Check sheet for the modelled part. Datum: model origin and axes. Units: mm. Face numbers are marked on the shaded views. Round coordinates to 2 decimals unless told otherwise and drop trailing zeros. Order: outer loops, then holes, each group sorted by start corner. A loop starts at its lowest first (then second) coordinate and runs counter-clockwise, first axis right, second up.
Q1. Cross-section at D-D on y = 2.5. Give the number of separate pieces and of enclosed holes in the cut face, then the cut area to 3 significant figures.
Q2. Cross-section at B-B on z = 9. Record the cut outline in (x, y), then the cut area to 3 significant figures.
Q3. Cross-section at C-C on z = 0. Record the cut outline in (x, y), then the cut area to 3 significant figures.
Q4. Mould release check, pull along Z, two halves, no side actions. Record for the marked faces 1, 2 and 3: +Z half, -Z half, draft (parallel to the pull), parting line (faces both ways), or undercut.
Q5. Depth check by flat-ended pin: P1, Ø3, axis at x = -1.5, z = -7, coming from the +Y side; P2, Ø4.5, axis at x = 12.12, z = -7, coming from the +Y side. Enter the tip coordinate at first touch or a pass-through.
Q6. Cross-section at A-A on x = -22.5. Record the cut outline in (y, z), then the cut area to 3 significant figures.
Q7. Scan lines: probe 1 along X at (y, z) = (3.8, -9); probe 2 along Z at (x, y) = (22.5, 3.85); probe 3 along X at (y, z) = (1, 14). Record each from-to range of solid material in increasing order.
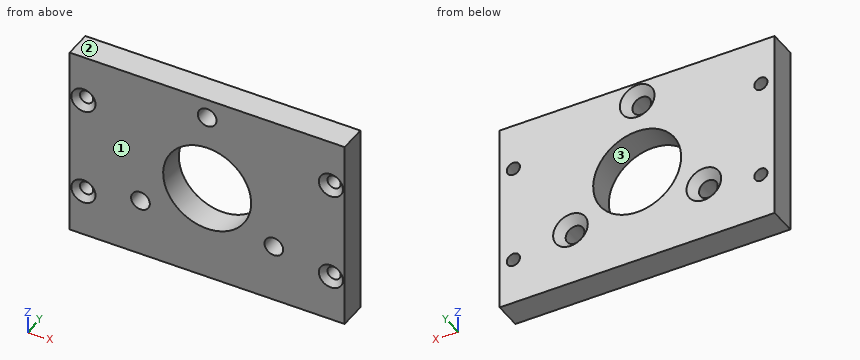
from build123d import *

# Parameters (mm, degrees)
SKETCH1_W                                           = 50
SKETCH1_H                                           = 35
SKETCH1_R                                           = 8
BOSS_EXTRUDE1_DEPTH                                 = 5
CSK_FOR_M3_COUNTERSUNK_FLAT_HEAD_SCREW1_D           = 3.4
CSK_FOR_M3_COUNTERSUNK_FLAT_HEAD_SCREW1_CSINK_D     = 6.3
CSK_FOR_M3_COUNTERSUNK_FLAT_HEAD_SCREW1_CSINK_ANGLE = 90
CSK_FOR_M2_COUNTERSUNK_FLAT_HEAD_SCREW1_D           = 2.4
CSK_FOR_M2_COUNTERSUNK_FLAT_HEAD_SCREW1_CSINK_D     = 4.4
CSK_FOR_M2_COUNTERSUNK_FLAT_HEAD_SCREW1_CSINK_ANGLE = 90


with BuildPart() as part:
    # Sketch1 → Boss-Extrude1 (new body)
    with BuildSketch(Plane(origin=(0, 0, 0), x_dir=(1, 0, 0), z_dir=(0, 1, 0))):
        Rectangle(SKETCH1_W, SKETCH1_H)
        with Locations(Location((0, 0, 0), (0, 0, 270))):
            Circle(SKETCH1_R, mode=Mode.SUBTRACT)
    extrude(amount=BOSS_EXTRUDE1_DEPTH)

    # CSK for M3 Countersunk Flat Head Screw1 (through all)
    with Locations(Plane(origin=(0, 5, 0), x_dir=(1, 0, 0), z_dir=(0, 1, 0))):
        with Locations((12.124355653, 7), (0, -14), (-12.124355653, 7)):
            CounterSinkHole(CSK_FOR_M3_COUNTERSUNK_FLAT_HEAD_SCREW1_D / 2, CSK_FOR_M3_COUNTERSUNK_FLAT_HEAD_SCREW1_CSINK_D / 2, counter_sink_angle=CSK_FOR_M3_COUNTERSUNK_FLAT_HEAD_SCREW1_CSINK_ANGLE)

    # CSK for M2 Countersunk Flat Head Screw1 (through all)
    with Locations(Plane(origin=(0, 0, 0), x_dir=(-1, 0, 0), z_dir=(0, -1, 0))):
        with Locations((22.5, -9), (22.5, 9), (-22.5, 9), (-22.5, -9)):
            CounterSinkHole(CSK_FOR_M2_COUNTERSUNK_FLAT_HEAD_SCREW1_D / 2, CSK_FOR_M2_COUNTERSUNK_FLAT_HEAD_SCREW1_CSINK_D / 2, counter_sink_angle=CSK_FOR_M2_COUNTERSUNK_FLAT_HEAD_SCREW1_CSINK_ANGLE)


solid = part.part
Results found:
1. separate pieces: 1
1. enclosed holes: 8
1. area: 1,500 mm2
2. outline: (-25, 0) - (-24.7, 0) - (-23.7, 1) - (-23.7, 5) - (-25, 5) - close; (-21.3, 1) - (-20.3, 0) - (20.3, 0) - (21.3, 1) - (21.3, 5) - (-21.3, 5) - close; (23.7, 1) - (24.7, 0) - (25, 0) - (25, 5) - (23.7, 5) - close
2. area: 224 mm2
3. outline: (-25, 0) - (-8, 0) - (-8, 5) - (-25, 5) - close; (8, 0) - (25, 0) - (25, 5) - (8, 5) - close
3. area: 170 mm2
4. face 1: draft
4. face 2: +Z half
4. face 3: undercut
5. P1: stops at y = 5
5. P2: stops at y = 4.1
6. outline: (0, -17.5) - (5, -17.5) - (5, -10.2) - (1, -10.2) - (0, -11.2) - close; (0, -6.8) - (1, -7.8) - (5, -7.8) - (5, 7.8) - (1, 7.8) - (0, 6.8) - close; (0, 11.2) - (1, 10.2) - (5, 10.2) - (5, 17.5) - (0, 17.5) - close
6. area: 149 mm2
7. probe 1: x = -25 to -23.7, -21.3 to 21.3, 23.7 to 25
7. probe 2: z = -17.5 to -10.2, -7.8 to 7.8, 10.2 to 17.5
7. probe 3: x = -25 to -1.7, 1.7 to 25
